The model under review builds one solid part; all positions refer to its coordinate system, in mm. A direction names the side the tool comes from. Coordinates: 2 decimals unless noted, no trailing zeros. Loops run counter-clockwise (first coordinate to the right, second up) from the corner with the lowest first, then second, coordinate; pieces in that order, holes last. Notation, with made-up numbers: M 30,67.25 L 57,67.25 A28 ccw 57,100.25 Z; hole C 35.5,7.25 d11. An arc over 180 degrees is marked long. One line per item, written item: value.
```python
from build123d import *

# Parameters (mm, degrees)
SKETCH_1_R          = 2.525444103
SKETCH_1_R_2        = 1.206738485
EXTRUDE_1_DEPTH     = 15
EXTRUDE_1_2_DEPTH   = 15
EXTRUDE_1_3_DEPTH   = 15
EXTRUDE_1_4_DEPTH   = 15
EXTRUDE_2_DEPTH     = 1
SKETCH_3_R          = 1.206738485
EXTRUDE_3_DEPTH     = 9
EXTRUDE_4_DEPTH     = 5
EXTRUDE_START       = 20
EXTRUDE_5_DEPTH     = 20
CUT_EXTRUDE_1_DEPTH = 2
FILLET_1_R          = 0.5
SKETCH_7_R          = 14.601754061
SKETCH_7_R_2        = 8.492985931
EXTRUDE_6_DEPTH     = 2
SKETCH_8_R          = 34
EXTRUDE_7_DEPTH     = 25


with BuildPart() as part:
    # Sketch 1 → Extrude 1 (new body)
    with BuildSketch(Plane(origin=(0, 0, 0), x_dir=(1, 0, 0), z_dir=(0, 1, 0))):
        with Locations(Location((-28.387774848, 41.175361777, 0), (0, 0, 270))):
            Circle(SKETCH_1_R)
        with Locations(Location((-28.387774848, 41.175361777, 0), (0, 0, 270))):
            Circle(SKETCH_1_R_2, mode=Mode.SUBTRACT)
    extrude(amount=EXTRUDE_1_DEPTH)



with BuildPart() as body_2:
    # Sketch 1 → Extrude 1 2 (new body)
    with BuildSketch(Plane(origin=(0, 0, 0), x_dir=(1, 0, 0), z_dir=(0, 1, 0))):
        with Locations(Location((27.718646552, 41.175361777, 0), (0, 0, 270))):
            Circle(SKETCH_1_R)
        with Locations(Location((27.718646552, 41.175361777, 0), (0, 0, 270))):
            Circle(SKETCH_1_R_2, mode=Mode.SUBTRACT)
    extrude(amount=EXTRUDE_1_2_DEPTH)


with BuildPart() as body_3:
    # Sketch 1 → Extrude 1 3 (new body)
    with BuildSketch(Plane(origin=(0, 0, 0), x_dir=(1, 0, 0), z_dir=(0, 1, 0))):
        with Locations(Location((19.695499635, -28.946408229, 0), (0, 0, 270))):
            Circle(SKETCH_1_R)
        with Locations(Location((19.695499635, -28.946408229, 0), (0, 0, 270))):
            Circle(SKETCH_1_R_2, mode=Mode.SUBTRACT)
    extrude(amount=EXTRUDE_1_3_DEPTH)


with BuildPart() as body_4:
    # Sketch 1 → Extrude 1 4 (new body)
    with BuildSketch(Plane(origin=(0, 0, 0), x_dir=(1, 0, 0), z_dir=(0, 1, 0))):
        with Locations(Location((-20.384564295, -29.006371883, 0), (0, 0, 270))):
            Circle(SKETCH_1_R)
        with Locations(Location((-20.384564295, -29.006371883, 0), (0, 0, 270))):
            Circle(SKETCH_1_R_2, mode=Mode.SUBTRACT)
    extrude(amount=EXTRUDE_1_4_DEPTH)


with BuildPart() as part_1:
    add(part.part)

    add(body_2.part)  # Extrude 2 merges body 2

    add(body_3.part)  # Extrude 2 merges body 3

    add(body_4.part)  # Extrude 2 merges body 4
    # Sketch 2 → Extrude 2 (add)
    with BuildSketch(Plane(origin=(0, 15, 0), x_dir=(1, 0, 0), z_dir=(0, 1, 0))):
        with BuildLine():
            ThreePointArc((-0.271405212, 48.428059813), (-15.076874658, 47.395350678), (-29.591025821, 44.295700747))
            ThreePointArc((-29.591025821, 44.295700747), (-30.425446284, 43.813362835), (-30.937389258, 42.996771284))
            ThreePointArc((-30.937389258, 42.996771284), (-35.014604001, 5.325002623), (-23.460887401, -30.7623562))
            ThreePointArc((-23.460887401, -30.7623562), (-20.186933133, -32.543063374), (-17.131754901, -30.40868277))
            ThreePointArc((-17.131754901, -30.40868277), (-15.675739537, -28.10111065), (-13.582203175, -26.351260562))
            ThreePointArc((-13.582203175, -26.351260562), (-0.271405212, -22.664793676), (13.039392752, -26.351260562))
            ThreePointArc((13.039392752, -26.351260562), (15.132929113, -28.10111065), (16.588944478, -30.40868277))
            ThreePointArc((16.588944478, -30.40868277), (19.644122709, -32.543063374), (22.918076977, -30.7623562))
            ThreePointArc((22.918076977, -30.7623562), (34.471793578, 5.325002623), (30.394578834, 42.996771284))
            ThreePointArc((30.394578834, 42.996771284), (29.88263586, 43.813362835), (29.048215398, 44.295700747))
            ThreePointArc((29.048215398, 44.295700747), (14.534064235, 47.395350678), (-0.271405212, 48.428059813))
        make_face()
    extrude(amount=EXTRUDE_2_DEPTH)

    # Sketch 3 → Extrude 3 (add)
    # profile 1 of 4: a face of its own
    with BuildSketch(Plane(origin=(0, 16, 0), x_dir=(1, 0, 0), z_dir=(0, 1, 0))):
        Polygon((22.207746053, -29.204256732), (21.174926198, -26.899663262), (18.66267978, -26.641814759), (17.183253217, -28.688559726), (18.216073072, -30.993153196), (20.72831949, -31.251001699), align=None)
        with Locations(Location((19.695499635, -28.946408229, 0), (0, 0, 270))):
            Circle(SKETCH_3_R, mode=Mode.SUBTRACT)
    # profile 2 of 4: a face of its own
    with BuildSketch(Plane(origin=(0, 16, 0), x_dir=(1, 0, 0), z_dir=(0, 1, 0))):
        Polygon((-18.905137732, -26.959626916), (-21.41738415, -26.701778413), (-22.896810713, -28.74852338), (-21.863990858, -31.05311685), (-19.35174444, -31.310965353), (-17.872317877, -29.264220386), align=None)
        with Locations(Location((-20.384564295, -29.006371883, 0), (0, 0, 270))):
            Circle(SKETCH_3_R, mode=Mode.SUBTRACT)
    # profile 3 of 4: a face of its own
    with BuildSketch(Plane(origin=(0, 16, 0), x_dir=(1, 0, 0), z_dir=(0, 1, 0))):
        Polygon((26.685826697, 43.479955247), (25.206400134, 41.43321028), (26.239219989, 39.12861681), (28.751466407, 38.870768307), (30.23089297, 40.917513274), (29.198073115, 43.222106744), align=None)
        with Locations(Location((27.718646552, 41.175361777, 0), (0, 0, 270))):
            Circle(SKETCH_3_R, mode=Mode.SUBTRACT)
    # profile 4 of 4: a face of its own
    with BuildSketch(Plane(origin=(0, 16, 0), x_dir=(1, 0, 0), z_dir=(0, 1, 0))):
        Polygon((-30.900021266, 41.43321028), (-29.867201411, 39.12861681), (-27.354954993, 38.870768307), (-25.87552843, 40.917513274), (-26.908348285, 43.222106744), (-29.420594703, 43.479955247), align=None)
        with Locations(Location((-28.387774848, 41.175361777, 0), (0, 0, 270))):
            Circle(SKETCH_3_R, mode=Mode.SUBTRACT)
    extrude(amount=EXTRUDE_3_DEPTH)

    # Sketch 4 → Extrude 4 (add)
    with BuildSketch(Plane(origin=(0, 25, 0), x_dir=(1, 0, 0), z_dir=(0, 1, 0))):
        with BuildLine():
            ThreePointArc((-0.271405212, 48.428034147), (-15.594215434, 47.321055953), (-30.593831711, 44.000600361))
            ThreePointArc((-30.593831711, 44.000600361), (-35.27623055, 8.446713655), (-25.910625184, -26.169599767))
            ThreePointArc((-25.910625184, -26.169599767), (-18.523285067, -36.56455338), (-8.301229723, -44.18934447))
            ThreePointArc((-8.301229723, -44.18934447), (-0.271405212, -46.17502358), (7.758419299, -44.18934447))
            ThreePointArc((7.758419299, -44.18934447), (17.980474644, -36.56455338), (25.36781476, -26.169599767))
            ThreePointArc((25.36781476, -26.169599767), (34.733420126, 8.446713655), (30.051021288, 44.000600361))
            ThreePointArc((30.051021288, 44.000600361), (15.05140501, 47.321055953), (-0.271405212, 48.428034147))
        make_face()
    extrude(amount=EXTRUDE_4_DEPTH)

    # Sketch 5 → Extrude 5 (add)
    with BuildSketch(Plane.XZ.offset(-25).offset(EXTRUDE_START)):
        with BuildLine():
            ThreePointArc((15.323487668, 36.26928355), (-0.271405212, 46.17502358), (-15.866298092, 36.26928355))
            ThreePointArc((-15.866298092, 36.26928355), (-16.212731749, 30.227590505), (-12.285634009, 25.623247505))
            ThreePointArc((-12.285634009, 25.623247505), (-0.271405212, 22.664793676), (11.742823586, 25.623247505))
            ThreePointArc((11.742823586, 25.623247505), (15.669921326, 30.227590505), (15.323487668, 36.26928355))
        make_face()
    extrude(amount=-EXTRUDE_5_DEPTH)

    # Sketch 6 → Cut-Extrude 1 (cut)
    with BuildSketch(Plane.XZ.offset(-5)):
        with BuildLine():
            Line((-15.724205973, 36.56455338), (-13.8705587, 36.56455338))
            ThreePointArc((-13.8705587, 36.56455338), (-0.271405212, 44.534003013), (13.327748276, 36.56455338))
            Line((13.327748276, 36.56455338), (15.18139555, 36.56455338))
            ThreePointArc((15.18139555, 36.56455338), (-0.271405212, 46.17502358), (-15.724205973, 36.56455338))
        make_face()
    extrude(amount=-CUT_EXTRUDE_1_DEPTH, mode=Mode.SUBTRACT)

    # Fillet 1
    fillet_1_edges = [part_1.edges().sort_by_distance(p)[0] for p in [
        (-0.271405212, 7, 46.17502358),
    ]]
    fillet(fillet_1_edges, radius=FILLET_1_R)

    # Sketch 7 → Extrude 6 (add)
    with BuildSketch(Plane(origin=(0, 30, 0), x_dir=(1, 0, 0), z_dir=(0, 1, 0))):
        with Locations(Location((-0.271405212, 14.438151783, 0), (0, 0, 270))):
            Circle(SKETCH_7_R)
        with Locations(Location((-0.271405212, -30.637034449, 0), (0, 0, 270))):
            Circle(SKETCH_7_R_2)
    extrude(amount=EXTRUDE_6_DEPTH)

    # Sketch 8 → Extrude 7 (add)
    with BuildSketch(Plane(origin=(0, 32, 0), x_dir=(1, 0, 0), z_dir=(0, 1, 0))):
        with Locations(Location((-0.271405212, 14.438151783, 0), (0, 0, 270))):
            Circle(SKETCH_8_R)
    extrude(amount=EXTRUDE_7_DEPTH)


solid = part_1.part
```
(1) Add section B-B on z = -35.5. State the section outline as (x, y) points.
Checks:
outline: M -33.04,15 L 32.5,15 L 32.5,16 L -33.04,16 Z; M -33.04,25 L 32.5,25 L 32.5,30 L -33.04,30 Z; M -26.96,32 L 26.42,32 L 26.42,57 L -26.96,57 Z
(2) Add section A-A on y = 12.5. State how many separate pieces and enclosed holes the cut face has, then the cut area to 3 significant figures.
Checks:
separate pieces: 5
enclosed holes: 4
area: 660 mm^2
(3) Insertion check: pin 1 Ø1.2 at (x, z) = (19.5, 28.5) entering from -Y; pin 2 Ø1.5 at (x, y) = (11, 29) entering from +Z; pin 3 Ø1.5 at (x, y) = (-1, 51) entering from +Z. Each pin has a flat end and moves straight along its axis. Give the tip position at first contact, or say it passes through.
Checks:
pin 1: y = 15
pin 2: z = 42.76
pin 3: z = 19.56
(4) Add section D-D on z = 16. State the section outline as (x, y) points, then the cut area to 3 significant figures.
Checks:
outline: M -30.23,15 L 29.68,15 L 29.68,16 L -30.23,16 Z; M -30.23,25 L 29.68,25 L 29.68,30 L -30.23,30 Z; M -15.42,32 L 14.88,32 L 14.88,57 L -15.42,57 Z
area: 1,120 mm^2
(5) To check wall thickness, follow L1, parallel to Y at x = 9.5, z = 1; L2, parallel to Y at x = -31, z = 2.5; L3, parallel to X at y = 10, z = -43.5. State the ranges of each line that lie inside material, in increasing order. Write a range as [from, to].
Checks:
L1: [15, 16], [25, 30], [32, 57]
L2: [15, 16], [25, 30]
L3: [-29.37, -27.4], [26.73, 28.71]
(6) Tool access review of faces 1 (the face through (-1, 5, 34)), 2 (the face through (-30.15, 20.44, -42.47)), 3 (the face through (21.825, 7.395, 30.304)): name each direction out of +Z, -Z, +X, -X, +Y, -Y from which nothing blocks a thin tool from reaching the whole face with its end or side.
Checks:
face 1: +Z, -Z, -Y
face 2: -Z, -X
face 3: -Y
(7) Add section C-C on z = -4. State the section outline as (x, y) points, then the cut area to 3 significant figures.
Checks:
outline: M -34.87,15 L 34.33,15 L 34.33,16 L -34.87,16 Z; M -34.87,25 L 34.33,25 L 34.33,30 L 9.94,30 L 9.94,32 L 32.09,32 L 32.09,57 L -32.63,57 L -32.63,32 L -10.48,32 L -10.48,30 L -34.87,30 Z
area: 2,070 mm^2
(8) Draft analysis for pull direction Z (two halves, no side actions). For faces 4 (the face through (30.223, 7.395, -41.504)), 5 (the face through (-20, 15, 29)), 6 (the face through (28, 16, -41)), 7 (the face through (17.69, 20.44, 29.82)), state which applies: pulls with the +Z half, pulls with the -Z half, needs draft (parallel to the pull), parting line crosses it, or undercut.
Checks:
face 4: parting line crosses it
face 5: undercut
face 6: undercut
face 7: pulls with the +Z half
